The listing builds one solid part. Answer for the finished solid, in the listing's coordinates (mm). A direction names the side the tool comes from. Give positions to 0.01 mm unless a question says otherwise; leave off trailing zeros. Write each loop counter-clockwise with the first axis right and the second up, starting at its lowest first coordinate (ties: lowest second). Pieces come first, ordered by that corner, then holes. Notation, with made-up numbers: M -25,57 L 20,57 A24 ccw 20,92 Z; hole C -30,-36.75 d4. An arc over 180 degrees is marked long. Return JSON: item names as keys, results as strings.
from build123d import *

# Parameters (mm, degrees)
SKETCH1_W           = 41.858784395
SKETCH1_H           = 34.22014658
BOSS_EXTRUDE1_DEPTH = 34
FILLET1_R           = 1
FILLET2_R           = 5
FILLET3_R           = 5


with BuildPart() as part:
    # Sketch1 → Boss-Extrude1 (new body)
    with BuildSketch(Plane.XY):
        Polygon((23.981900452, 10.610859729), (-16.018099548, 10.610859729), (-18.518099548, 10.610859729), (-18.518099548, -9.389140271), (-21.018099548, -29.389140271), (-76.018099548, -29.389140271), (-76.018099548, 10.610859729), (-76.018099548, 15.610859729), (13.981900452, 15.610859729), (13.981900452, 35.610859729), (23.981900452, 35.610859729), (23.981900452, 15.610859729), align=None)
        with Locations((-48.518099548, -6.499213561)):
            Rectangle(SKETCH1_W, SKETCH1_H, mode=Mode.SUBTRACT)
    extrude(amount=BOSS_EXTRUDE1_DEPTH)

    # Fillet1
    fillet1_edges = [part.edges().sort_by_distance(p)[0] for p in [
        (-18.518099548, 10.610859729, 17),
        (13.981900452, 15.610859729, 17),
    ]]
    fillet(fillet1_edges, radius=FILLET1_R)

    # Fillet2
    fillet2_edges = [part.edges().sort_by_distance(p)[0] for p in [
        (-27.58870735, 10.610859729, 17),
        (-69.447491745, 10.610859729, 17),
        (-69.447491745, -23.609286851, 17),
        (-27.58870735, -23.609286851, 17),
    ]]
    fillet(fillet2_edges, radius=FILLET2_R)

    # Fillet3
    fillet3_edges = [part.edges().sort_by_distance(p)[0] for p in [
        (13.981900452, 35.610859729, 17),
        (23.981900452, 35.610859729, 17),
        (23.981900452, 10.610859729, 17),
        (-76.018099548, 15.610859729, 17),
        (-76.018099548, -29.389140271, 17),
        (-21.018099548, -29.389140271, 17),
    ]]
    fillet(fillet3_edges, radius=FILLET3_R - 0.0001)  # a hair under: the kernel refuses the full size


solid = part.part
Item 1: Which of the six approach directions +Z, -Z, +X, -X, +Y, -Y give full straight-line access (tool end or side, diameter ignored) to faces 1 (the flat face through (-30, 15.611, 17)), 2 (the flat face through (-49, 10.611, 17)), 3 (the flat face through (0, 10.611, 17))?
Geometry results:
{"face 1": "+Z, -Z, -X, +Y", "face 2": "+Z, -Z", "face 3": "+Z, -Z, +X, -Y"}
Item 2: Given pin 1 Ø5.5 at (y, z) = (4, 24.5) entering from +X; pin 2 Ø2 at (x, z) = (-24.5, 15.5) entering from +Y; pin 3 Ø10 at (x, z) = (8.5, 13) entering from -Y, each flat-ended and moving along its own axis, determine where each tip first touches the part or whether it passes through.
Geometry results:
{"pin 1": "stops at x = -18.52", "pin 2": "stops at y = 15.61", "pin 3": "stops at y = 10.61"}
Item 3: Determine the mould class of faces 4 (the cylindrical face through (-74.515, -27.963, 17.238)), 5 (the cylindrical face through (-29.015, -22.106, 17.238)), 6 (the cylindrical face through (15.5, 34.2, 17.2)) for opening direction Y: +Y half, -Y half, draft (parallel to the pull), parting line (faces both ways), or undercut.
Geometry results:
{"face 4": "-Y half", "face 5": "undercut", "face 6": "+Y half"}
Item 4: A cutting plane is placed at B-B, the plane y = -4. Write down the section's boundary in (x, z), plus the area to 3 significant figures.
Geometry results:
{"outline": "M -76.02,0 L -69.45,0 L -69.45,34 L -76.02,34 Z; M -27.59,0 L -18.52,0 L -18.52,34 L -27.59,34 Z", "area": "532 mm2"}
Item 5: Find the intervals of material crossed by line 1 (X direction, y = -8, z = 3.5); line 2 (Y direction, x = -41, z = 10); line 3 (Y direction, x = 4, z = 3.5), in increasing order.
Geometry results:
{"line 1": "x = -76.02 to -69.45, -27.59 to -18.52", "line 2": "y = -29.39 to -23.61, 10.61 to 15.61", "line 3": "y = 10.61 to 15.61"}
Item 6: A cutting plane is placed at D-D, the plane y = 21. Write down the section's boundary in (x, z), plus the area to 3 significant figures.
Geometry results:
{"outline": "M 13.98,0 L 23.98,0 L 23.98,34 L 13.98,34 Z", "area": "340 mm2"}
Item 7: A cutting plane is placed at C-C, the plane x = -54. Write down the section's boundary in (y, z).
Geometry results:
{"outline": "M -29.39,0 L -23.61,0 L -23.61,34 L -29.39,34 Z; M 10.61,0 L 15.61,0 L 15.61,34 L 10.61,34 Z"}
